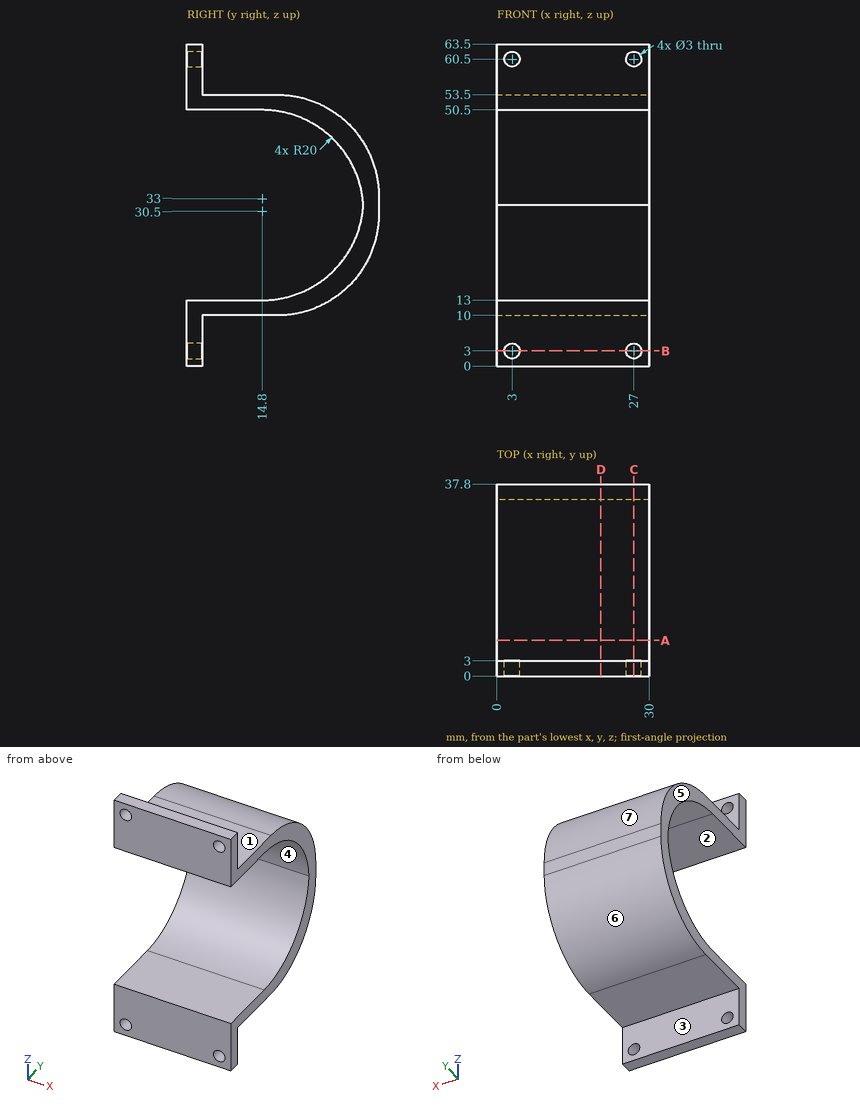
Geometry check sheet. Reference: drawing and pictorial views, mm from the part's lowest x, y, z. A direction names the side the tool comes from. Give positions to 0.01 mm unless a question says otherwise; leave off trailing zeros. Order: outer loops, then holes, each group sorted by start corner. A loop starts at its lowest first (then second) coordinate and runs counter-clockwise, first axis right, second up. Notation, with made-up numbers: M -28.5,14 L 15.5,14 A13 ccw 15.5,25 Z; hole C 18.5,17 d5. An arc over 180 degrees is marked long. Answer in a Markdown table with one row per item. Add a question column.
Item 1: Tool access check on the marked faces 1, 2 and 3. Record the directions out of +Z, -Z, +X, -X, +Y, -Y that give a thin tool (end or side, any length) a straight path to the whole face; none if there is none.
Item 2: Section check D-D, the plane x = 20.5. Enter the section's corners in (y, z), and give its area (3 significant figures).
Item 3: Section check A-A, the plane y = 7. Enter the section's corners in (x, z), and give its area (3 significant figures).
Item 4: Gauge pin test, flat ends, axial feed: pin 1 (3 mm diameter, centred on x = 21, z = 57, fed in from +Y); pin 2 (12 mm diameter, centred on x = 15.5, y = 18.5, fed in from +Z); pin 3 (10 mm diameter, centred on x = 11, z = 10, fed in from +Y); pin 4 (1.8 mm diameter, centred on x = 27, z = 60.5, fed in from -Y). Record the tip position at first contact, or that the pin passes through.
Item 5: Scan lines: probe 1 along Z at (x, y) = (19, 14.5); probe 2 along Y at (x, z) = (24, 4); probe 3 along Z at (x, y) = (11, 28). Record each from-to range of solid material in increasing order. Write a range as from..to.
Item 6: Section check C-C, the plane x = 27. Enter the section's corners in (y, z), and give its area (3 significant figures).
Item 7: Section check B-B, the plane z = 3. Enter the section's corners in (x, y), and give its area (3 significant figures).
Item 8: Mould release check, pull along Z, two halves, no side actions. Record for the marked faces 4, 5, 6 and 7: released by +Z, released by -Z, zero draft, split by the parting line, or undercut.
Filled sheet:
| question | item | result |
|---|---|---|
| 1 | face 1 | +Z, +X, -X, +Y |
| 1 | face 2 | +X, -X, -Y |
| 1 | face 3 | -Z, +X, -X, +Y |
| 2 | outline | M 0,0 L 3,0 L 3,10 L 17.8,10 A20 ccw 37.8,30 L 37.8,33.5 A20 ccw 17.8,53.5 L 3,53.5 L 3,63.5 L 0,63.5 L 0,50.5 L 14.8,50.5 A20 cw 34.76,31.75 A20 cw 14.8,13 L 0,13 Z |
| 2 | area | 399 mm^2 |
| 3 | outline | M 0,10 L 30,10 L 30,13 L 0,13 Z; M 0,50.5 L 30,50.5 L 30,53.5 L 0,53.5 Z |
| 3 | area | 180 mm^2 |
| 4 | pin 1 | stops at y = 3 |
| 4 | pin 2 | stops at z = 53.5 |
| 4 | pin 3 | stops at y = 31.03 |
| 4 | pin 4 | passes through |
| 5 | probe 1 | z = 10..13, 50.5..53.5 |
| 5 | probe 2 | y = 0..3 |
| 5 | probe 3 | z = 12.8..17.97, 45.53..50.7 |
| 6 | outline | M 0,0 L 3,0 L 3,1.5 L 0,1.5 Z; M 0,4.5 L 3,4.5 L 3,10 L 17.8,10 A20 ccw 37.8,30 L 37.8,33.5 A20 ccw 17.8,53.5 L 3,53.5 L 3,59 L 0,59 L 0,50.5 L 14.8,50.5 A20 cw 34.76,31.75 A20 cw 14.8,13 L 0,13 Z; M 0,62 L 3,62 L 3,63.5 L 0,63.5 Z |
| 6 | area | 381 mm^2 |
| 7 | outline | M 0,0 L 1.5,0 L 1.5,3 L 0,3 Z; M 4.5,0 L 25.5,0 L 25.5,3 L 4.5,3 Z; M 28.5,0 L 30,0 L 30,3 L 28.5,3 Z |
| 7 | area | 72.0 mm^2 |
| 8 | face 4 | undercut |
| 8 | face 5 | zero draft |
| 8 | face 6 | released by -Z |
| 8 | face 7 | released by +Z |
